Here's the drawing with two shaded views (mm, measured from the low corner). I have some questions. Round coordinates to 2 decimals unless told otherwise and drop trailing zeros. Order: outer loops, then holes, each group sorted by start corner. A loop starts at its lowest first (then second) coordinate and runs counter-clockwise, first axis right, second up. Notation, with made-up numbers: (-19.5, 41.25) -> (6.5, 41.25) arc R29 cw to (6.5, 68.25) -> close; hole circle Ø5 at (-27, -12.75). An arc over 180 degrees is marked (long way). Use a Markdown table: item, result. Add a question column.
Q1. I'm going to push flat-ended pins straight in: pin 1 Ø5 at (x, y) = (15.5, 176.5) entering from +Z; pin 2 Ø1 at (x, z) = (24, 263.5) entering from +Y; pin 3 Ø5 at (x, y) = (22, 88.5) entering from +Z. Where does each tip first touch, or does it pass through?
Q2. If we section it at B-B on y = 153: List the corners of the cut face in (x, z) for me.
Q3. If we section it at D-D on z = 82: List the corners of the cut face in (x, y) for me (3 decimals).
Q4. I need wall thicknesses on line 1 along X through (y, z) = (5, 150); line 2 along Z through (x, y) = (28.5, 113); line 3 along Y through (x, z) = (9, 254.5). Which ranges of each line are inside material? Lowest first, please. Write a range as [from, to].
Q5. We'd pull the mould along Y, two halves only. Please class the marked faces 1 and 2: +Y half, -Y half, draft (parallel to the pull), parting line (faces both ways), or undercut.
Q6. If we section it at C-C on z = 260: List the corners of the cut face in (x, y) for me.
Q7. If we section it at A-A on x = 8: List the corners of the cut face in (y, z) for me, plus the area to 3 significant figures.
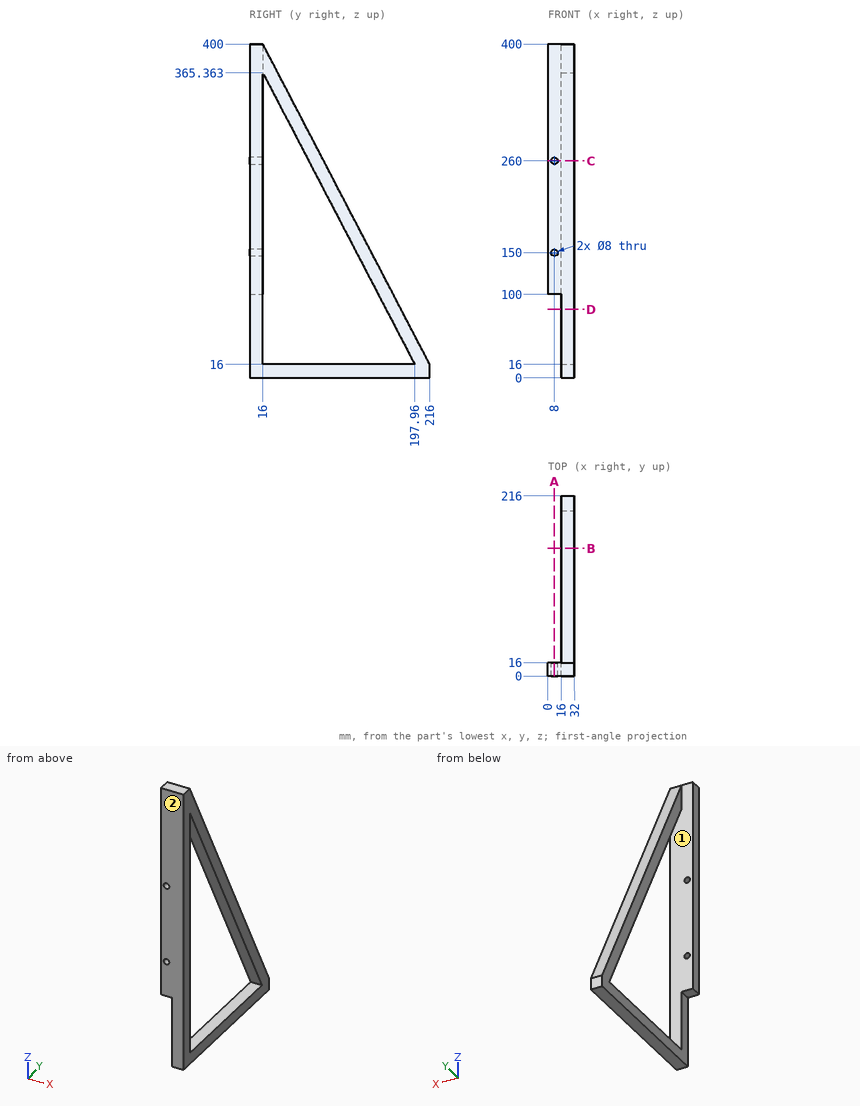
Answer below:
| question | item | result |
|---|---|---|
| 1 | pin 1 | z = 96.54 |
| 1 | pin 2 | y = 87.35 |
| 1 | pin 3 | z = 265.6 |
| 2 | outline | (16, 0) -> (32, 0) -> (32, 16) -> (16, 16) -> close; (16, 102.32) -> (32, 102.32) -> (32, 136.96) -> (16, 136.96) -> close |
| 3 | outline | (16, 0) -> (32, 0) -> (32, 16) -> (16, 16) -> close; (16, 163.585) -> (32, 163.585) -> (32, 181.625) -> (16, 181.625) -> close |
| 4 | line 1 | [0, 4], [12, 32] |
| 4 | line 2 | [0, 16], [179.12, 213.76] |
| 4 | line 3 | [0, 16] |
| 5 | face 1 | undercut |
| 5 | face 2 | -Y half |
| 6 | outline | (0, 0) -> (4, 0) -> (4, 16) -> (0, 16) -> close; (12, 0) -> (32, 0) -> (32, 16) -> (12, 16) -> close; (16, 70.88) -> (32, 70.88) -> (32, 88.92) -> (16, 88.92) -> close |
| 7 | outline | (0, 100) -> (16, 100) -> (16, 146) -> (0, 146) -> close; (0, 154) -> (16, 154) -> (16, 256) -> (0, 256) -> close; (0, 264) -> (16, 264) -> (16, 400) -> (0, 400) -> close |
| 7 | area | 4,540 mm² |
